Could you check a few things on this model? Use its own coordinates, in mm. A direction names the side the tool comes from. Round coordinates to 2 decimals unless told otherwise and drop trailing zeros. Order: outer loops, then holes, each group sorted by start corner. A loop starts at its lowest first (then second) coordinate and runs counter-clockwise, first axis right, second up. Notation, with made-up numbers: (4, 47) - (63, 47) arc R11 cw to (63, 61) - close; hole circle Ø4 at (80.5, 84). An arc over 180 degrees is marked (long way). Use one line per item in the form item = value.
from build123d import *

# Parameters (mm, degrees)
SKETCH1_W            = 150
SKETCH1_H            = 125
SKETCH1_R            = 45
BOSS_EXTRUDE2_DEPTH  = 75
SKETCH1_5_R          = 45
SKETCH1_5_R_2        = 26
BOSS_EXTRUDE3_DEPTH  = 70
SKETCH6_R            = 27.5
BOSS_EXTRUDE5_DEPTH  = 16
SKETCH7_R            = 17.5
BOSS_EXTRUDE6_DEPTH  = 10.5
SKETCH8_R            = 27.5
BOSS_EXTRUDE7_DEPTH  = 13.5
BOSS_EXTRUDE8_START  = 16
SKETCH9_R            = 27.5
BOSS_EXTRUDE8_DEPTH  = 16
BOSS_EXTRUDE9_START  = 10.5
SKETCH10_R           = 17.5
BOSS_EXTRUDE9_DEPTH  = 10.5
BOSS_EXTRUDE10_START = 13.5
SKETCH11_R           = 27.5
BOSS_EXTRUDE10_DEPTH = 13.5


with BuildPart() as part:
    # Sketch1 → Boss-Extrude2 (new body)
    with BuildSketch(Plane.XY):
        Rectangle(SKETCH1_W, SKETCH1_H)
        Circle(SKETCH1_R, mode=Mode.SUBTRACT)
    extrude(amount=BOSS_EXTRUDE2_DEPTH)

    # Sketch1_5 → Boss-Extrude3 (add)
    with BuildSketch(Plane.XY):
        Circle(SKETCH1_5_R)
        Circle(SKETCH1_5_R_2, mode=Mode.SUBTRACT)
    extrude(amount=BOSS_EXTRUDE3_DEPTH)

    # Sketch6 → Boss-Extrude5 (add)
    with BuildSketch(Plane(origin=(75, 0, 0), x_dir=(0, 0, -1), z_dir=(1, 0, 0))):
        with Locations((-37.5, 0)):
            Circle(SKETCH6_R)
    extrude(amount=BOSS_EXTRUDE5_DEPTH)

    # Sketch7 → Boss-Extrude6 (add)
    with BuildSketch(Plane(origin=(91, 0, 0), x_dir=(0, 0, -1), z_dir=(1, 0, 0))):
        with Locations(Location((-37.5, 0, 0), (0, 0, 180))):
            Circle(SKETCH7_R)
    extrude(amount=BOSS_EXTRUDE6_DEPTH)

    # Sketch8 → Boss-Extrude7 (add)
    with BuildSketch(Plane(origin=(101.5, 0, 0), x_dir=(0, 0, -1), z_dir=(1, 0, 0))):
        with Locations((-37.5, 0)):
            Circle(SKETCH8_R)
    extrude(amount=BOSS_EXTRUDE7_DEPTH)

    # Sketch9 → Boss-Extrude8 (add)
    with BuildSketch(Plane.ZY.offset(75).offset(BOSS_EXTRUDE8_START)):
        with Locations(Location((37.5, 0, 0), (0, 0, 180))):
            Circle(SKETCH9_R)
    extrude(amount=-BOSS_EXTRUDE8_DEPTH)

    # Sketch10 → Boss-Extrude9 (add)
    with BuildSketch(Plane.ZY.offset(91).offset(BOSS_EXTRUDE9_START)):
        with Locations((37.5, 0)):
            Circle(SKETCH10_R)
    extrude(amount=-BOSS_EXTRUDE9_DEPTH)

    # Sketch11 → Boss-Extrude10 (add)
    with BuildSketch(Plane.ZY.offset(101.5).offset(BOSS_EXTRUDE10_START)):
        with Locations(Location((37.5, 0, 0), (0, 0, 180))):
            Circle(SKETCH11_R)
    extrude(amount=-BOSS_EXTRUDE10_DEPTH)


solid = part.part
Item 1: Imagine slicing it at B-B on x = 0. Please give me the cut outline in (y, z), plus the area to 4 significant figures.
Found:
outline = (-62.5, 0) - (-26, 0) - (-26, 70) - (-45, 70) - (-45, 75) - (-62.5, 75) - close; (26, 0) - (62.5, 0) - (62.5, 75) - (45, 75) - (45, 70) - (26, 70) - close
area = 5,285 mm2
Item 2: If we mould it in two halves opening along X, with no side actions, what happens to faces 6 (the face through (75, -29, 37)), 7 (the face through (101.5, -18, 38)), 8 (the face through (-115, 0, 38)), 9 (the face through (82.888, -16.733, 59.323))? For each: released by +X, released by -X, zero draft, split by the parting line, or undercut.
Found:
face_6 = released by +X
face_7 = undercut
face_8 = released by -X
face_9 = zero draft
Item 3: For faces 1 (the face through (115, 0, 38)), 2 (the face through (96.176, 6.703, 53.666)), 3 (the face through (-83.112, -1.209, 64.973)), 4 (the face through (20.765, -39.923, 72.465)), 5 (the face through (108.156, -16.733, 59.323)), which set-ups out of +Z, -Z, +X, -X, +Y, -Y let a thin tool reach every point of the face, with its end or its side?
Found:
face_1 = +Z, -Z, +X, +Y, -Y
face_2 = none
face_3 = -X
face_4 = +Z
face_5 = +X
Item 4: Will these pins go through, and if not, where does the flat tip stop? P1, Ø5, axis at x = -79.5, y = 6, coming from the -Z side; P2, Ø6, axis at y = -19, z = 13.5, coming from the +X side; P3, Ø2, axis at y = 42.5, z = 23, coming from the -X side; P4, Ø2, axis at x = 55, y = -17, coming from the -Z side.
Found:
P1 = 10.22
P2 = 75
P3 = -75
P4 = 0
Item 5: I need wall thicknesses on L1, parallel to Y at x = 0, z = 25; L2, parallel to Y at x = 0, z = 71.5; L3, parallel to X at y = -34.5, z = 15. Which ranges of each line are inside material? Lowest first, please.
Found:
L1 = -62.5 to -26, 26 to 62.5
L2 = -62.5 to -45, 45 to 62.5
L3 = -75 to 75
Item 6: Imagine slicing it at A-A on z = 62. Please give me the cut outline in (x, y), plus the area to 3 significant figures.
Found:
outline = (-115, -12.49) - (-101.5, -12.49) - (-101.5, 12.49) - (-115, 12.49) - close; (-91, -12.49) - (-75, -12.49) - (-75, -62.5) - (75, -62.5) - (75, -12.49) - (91, -12.49) - (91, 12.49) - (75, 12.49) - (75, 62.5) - (-75, 62.5) - (-75, 12.49) - (-91, 12.49) - close; (101.5, -12.49) - (115, -12.49) - (115, 12.49) - (101.5, 12.49) - close; hole circle Ø52 at (0, 0)
area = 18,100 mm2
Item 7: Imagine slicing it at C-C on y = 22.5. Please give me the cut outline in (x, z), plus the area to 3 significant figures.
Found:
outline = (-115, 21.69) - (-101.5, 21.69) - (-101.5, 53.31) - (-115, 53.31) - close; (-91, 21.69) - (-75, 21.69) - (-75, 0) - (-13.03, 0) - (-13.03, 70) - (-38.97, 70) - (-38.97, 75) - (-75, 75) - (-75, 53.31) - (-91, 53.31) - close; (13.03, 0) - (75, 0) - (75, 21.69) - (91, 21.69) - (91, 53.31) - (75, 53.31) - (75, 75) - (38.97, 75) - (38.97, 70) - (13.03, 70) - close; (101.5, 21.69) - (115, 21.69) - (115, 53.31) - (101.5, 53.31) - close
area = 10,900 mm2
